from build123d import *

# Parameters (mm, degrees)
SKETCH1_W           = 558.8
SKETCH1_H           = 368.6625
SKETCH1_W_2         = 552.45
SKETCH1_H_2         = 362.3125
SKETCH1_W_3         = 3.175
SKETCH1_W_4         = 89.789
SKETCH1_W_5         = 89.15625
SKETCH1_W_6         = 88.26275
BOSS_EXTRUDE1_DEPTH = 3.175
SKETCH2_W           = 558.8
SKETCH2_H           = 368.6625
SKETCH2_W_2         = 552.45
SKETCH2_H_2         = 362.3125
SKETCH2_W_3         = 3.175
BOSS_EXTRUDE2_DEPTH = 162.9
SKETCH3_W           = 558.8
SKETCH3_H           = 368.6625
BOSS_EXTRUDE3_DEPTH = 45
CUT_EXTRUDE1_DEPTH  = 509.457524805
SKETCH5_R           = 3
CUT_EXTRUDE2_DEPTH  = 509.457524805
LPATTERN1_COUNT     = 3
LPATTERN1_PITCH     = 185.928
SKETCH6_R           = 3
CUT_EXTRUDE3_DEPTH  = 509.457524805
LPATTERN2_COUNT     = 2
LPATTERN2_PITCH     = 185.928


with BuildPart() as part:
    # Sketch1 → Boss-Extrude1 (new body)
    # profile 1 of 12: a face of its own
    with BuildSketch(Plane.XY):
        Rectangle(SKETCH1_W, SKETCH1_H)
        Rectangle(SKETCH1_W_2, SKETCH1_H_2, mode=Mode.SUBTRACT)
    # profile 2 of 12: a face of its own
    with BuildSketch(Plane.XY):
        with Locations((-185.48125, 0)):
            Rectangle(SKETCH1_W_3, SKETCH1_H_2)
    # profile 3 of 12: a face of its own
    with BuildSketch(Plane.XY):
        with Locations((-138.99925, 0)):
            Rectangle(SKETCH1_W_4, SKETCH1_H_2)
    # profile 4 of 12: a face of its own
    with BuildSketch(Plane.XY):
        with Locations((-231.646875, 0)):
            Rectangle(SKETCH1_W_5, SKETCH1_H_2)
    # profile 5 of 12: a face of its own
    with BuildSketch(Plane.XY):
        with Locations((-46.03525, 0)):
            Rectangle(SKETCH1_W_4, SKETCH1_H_2)
    # profile 6 of 12: a face of its own
    with BuildSketch(Plane.XY):
        with Locations((-92.51725, 0)):
            Rectangle(SKETCH1_W_3, SKETCH1_H_2)
    # profile 7 of 12: a face of its own
    with BuildSketch(Plane.XY):
        with Locations((46.92875, 0)):
            Rectangle(SKETCH1_W_4, SKETCH1_H_2)
    # profile 8 of 12: a face of its own
    with BuildSketch(Plane.XY):
        with Locations((0.44675, 0)):
            Rectangle(SKETCH1_W_3, SKETCH1_H_2)
    # profile 9 of 12: a face of its own
    with BuildSketch(Plane.XY):
        with Locations((139.89275, 0)):
            Rectangle(SKETCH1_W_4, SKETCH1_H_2)
    # profile 10 of 12: a face of its own
    with BuildSketch(Plane.XY):
        with Locations((93.41075, 0)):
            Rectangle(SKETCH1_W_3, SKETCH1_H_2)
    # profile 11 of 12: a face of its own
    with BuildSketch(Plane.XY):
        with Locations((232.093625, 0)):
            Rectangle(SKETCH1_W_6, SKETCH1_H_2)
    # profile 12 of 12: a face of its own
    with BuildSketch(Plane.XY):
        with Locations((186.37475, 0)):
            Rectangle(SKETCH1_W_3, SKETCH1_H_2)
    extrude(amount=BOSS_EXTRUDE1_DEPTH)

    # Sketch2 → Boss-Extrude2 (add)
    # profile 1 of 6: a face of its own
    with BuildSketch(Plane.XY.offset(3.175)):
        Rectangle(SKETCH2_W, SKETCH2_H)
        Rectangle(SKETCH2_W_2, SKETCH2_H_2, mode=Mode.SUBTRACT)
    # profile 2 of 6: a face of its own
    with BuildSketch(Plane.XY.offset(3.175)):
        with Locations((-185.48125, 0)):
            Rectangle(SKETCH2_W_3, SKETCH2_H_2)
    # profile 3 of 6: a face of its own
    with BuildSketch(Plane.XY.offset(3.175)):
        with Locations((-92.51725, 0)):
            Rectangle(SKETCH2_W_3, SKETCH2_H_2)
    # profile 4 of 6: a face of its own
    with BuildSketch(Plane.XY.offset(3.175)):
        with Locations((0.44675, 0)):
            Rectangle(SKETCH2_W_3, SKETCH2_H_2)
    # profile 5 of 6: a face of its own
    with BuildSketch(Plane.XY.offset(3.175)):
        with Locations((93.41075, 0)):
            Rectangle(SKETCH2_W_3, SKETCH2_H_2)
    # profile 6 of 6: a face of its own
    with BuildSketch(Plane.XY.offset(3.175)):
        with Locations((186.37475, 0)):
            Rectangle(SKETCH2_W_3, SKETCH2_H_2)
    extrude(amount=BOSS_EXTRUDE2_DEPTH)

    # Sketch3 → Boss-Extrude3 (add)
    with BuildSketch(Plane.XY.offset(166.075)):
        Rectangle(SKETCH3_W, SKETCH3_H)
        Polygon((187.96225, 181.15625), (276.225, 181.15625), (276.225, -181.15625), (187.96225, -181.15625), (184.78725, -181.15625), (94.99825, -181.15625), (91.82325, -181.15625), (2.03425, -181.15625), (-1.14075, -181.15625), (-90.92975, -181.15625), (-94.10475, -181.15625), (-183.89375, -181.15625), (-187.06875, -181.15625), (-276.225, -181.15625), (-276.225, 181.15625), (-187.06875, 181.15625), (-183.89375, 181.15625), (-94.10475, 181.15625), (-90.92975, 181.15625), (-1.14075, 181.15625), (2.03425, 181.15625), (91.82325, 181.15625), (94.99825, 181.15625), (184.78725, 181.15625), align=None, mode=Mode.SUBTRACT)
    extrude(amount=BOSS_EXTRUDE3_DEPTH)

    # Sketch4 → Cut-Extrude1 (cut, through all)
    with BuildSketch(Plane.XZ.offset(184.33125)):
        Polygon((279.4, 211.075), (209.4, 211.075), (279.4, 151.075), align=None)
    extrude(amount=-CUT_EXTRUDE1_DEPTH, mode=Mode.SUBTRACT)

    # Sketch5 → Cut-Extrude2 (cut, through all)
    with BuildSketch(Plane.XZ.offset(184.33125)):
        with Locations(Location((-210.146875, 12.7, 0), (0, 0, 270))):
            Circle(SKETCH5_R)
        with Locations(Location((-245.146875, 12.7, 0), (0, 0, 270))):
            Circle(SKETCH5_R)
        with Locations(Location((-210.146875, 132.7, 0), (0, 0, 270))):
            Circle(SKETCH5_R)
        with Locations(Location((-245.146875, 132.7, 0), (0, 0, 270))):
            Circle(SKETCH5_R)
    cut_extrude2 = extrude(amount=-CUT_EXTRUDE2_DEPTH, mode=Mode.SUBTRACT)

    # LPattern1: Cut-Extrude2 ×3
    with Locations(*[(i * LPATTERN1_PITCH, 0, 0) for i in range(1, LPATTERN1_COUNT)]):
        add(cut_extrude2, mode=Mode.SUBTRACT)

    # Sketch6 → Cut-Extrude3 (cut, through all)
    with BuildSketch(Plane.XZ.offset(184.33125)):
        with Locations(Location((-125.49925, 132.7, 0), (0, 0, 270))):
            Circle(SKETCH6_R)
        with Locations(Location((-160.49925, 132.7, 0), (0, 0, 270))):
            Circle(SKETCH6_R)
        with Locations(Location((-125.49925, 12.7, 0), (0, 0, 270))):
            Circle(SKETCH6_R)
        with Locations(Location((-160.49925, 12.7, 0), (0, 0, 270))):
            Circle(SKETCH6_R)
    cut_extrude3 = extrude(amount=-CUT_EXTRUDE3_DEPTH, mode=Mode.SUBTRACT)

    # LPattern2: Cut-Extrude3 ×2
    with Locations(*[(i * LPATTERN2_PITCH, 0, 0) for i in range(1, LPATTERN2_COUNT)]):
        add(cut_extrude3, mode=Mode.SUBTRACT)


solid = part.part
Work out the finished part from the listing and answer in its coordinate system (mm). A direction names the side the tool comes from. Coordinates: 2 decimals unless noted, no trailing zeros. Order: outer loops, then holes, each group sorted by start corner. A loop starts at its lowest first (then second) coordinate and runs counter-clockwise, first axis right, second up. Notation, with made-up numbers: (-37.75, 14) - (-12.75, 14) arc R22 ccw to (-12.75, 50) - close; hole circle Ø5 at (37, 21.25). An arc over 180 degrees is marked (long way). Put each result on its own line as item: value. Start each with the question number.
1) Find section A-A (z = 123). Give the vertices of the cut face in (x, y) (3 decimals).
2) Find section C-C (x = -149.5). Give the vertices of the cut face in (y, z) (3 decimals).
3) Flat-ended cylindrical pins translate along their axes: pin 1 (6 mm diameter, centred on x = -156.5, y = -118, fed in from -Z); pin 2 (5.5 mm diameter, centred on x = 126.71, z = 12.7, fed in from -Y); pin 3 (3.5 mm diameter, centred on x = -0.5, y = 22, fed in from +Z) (3 decimals). Find the tip coordinate at first contact, or state that the pin passes through.
4) Find section B-B (y = 29). Give the vertices of the cut face in (x, z) (3 decimals), plus the area to 3 significant figures.
5) Find the intervals of material crossed by line 1 (Y direction, x = 12, z = 139.5); line 2 (Z direction, x = -185, y = 122.5) (3 decimals); line 3 (Z direction, x = -251.5, y = -137) (3 decimals), in increasing order. Write a range as from..to.
6) For faces 4 (the flat face through (-90.93, -3, 83)), 5 (the flat face through (277.94, -0.86, 152.326)), determine the directions among +Z, -Z, +X, -X, +Y, -Y from which every point of the face is accessible in a straight line to the end or side of a thin tool.
7) For a pull along Y with two mould halves and no side action, classify faces 1 (the flat face through (-4, -184.331, 104)), 2 (the flat face through (-4, 181.156, 106)), 3 (the flat face through (-279.4, -3, 104)) as released by +Y, released by -Y, zero draft, split by the parting line, or undercut.
Results list:
1. outline: (-279.4, -184.331) - (279.4, -184.331) - (279.4, 184.331) - (-279.4, 184.331) - close; hole (-276.225, -181.156) - (-187.069, -181.156) - (-187.069, 181.156) - (-276.225, 181.156) - close; hole (-183.894, -181.156) - (-94.105, -181.156) - (-94.105, 181.156) - (-183.894, 181.156) - close; hole (-90.93, -181.156) - (-1.141, -181.156) - (-1.141, 181.156) - (-90.93, 181.156) - close; hole (2.034, -181.156) - (91.823, -181.156) - (91.823, 181.156) - (2.034, 181.156) - close; hole (94.998, -181.156) - (184.787, -181.156) - (184.787, 181.156) - (94.998, 181.156) - close; hole (187.962, -181.156) - (276.225, -181.156) - (276.225, 181.156) - (187.962, 181.156) - close
2. outline: (-184.331, 0) - (184.331, 0) - (184.331, 211.075) - (181.156, 211.075) - (181.156, 3.175) - (-181.156, 3.175) - (-181.156, 211.075) - (-184.331, 211.075) - close
3. pin 1: stops at z = 0
3. pin 2: passes through
3. pin 3: stops at z = 166.075
4. outline: (-279.4, 0) - (279.4, 0) - (279.4, 151.075) - (276.225, 153.796) - (276.225, 3.175) - (187.962, 3.175) - (187.962, 166.075) - (184.787, 166.075) - (184.787, 3.175) - (94.998, 3.175) - (94.998, 166.075) - (91.823, 166.075) - (91.823, 3.175) - (2.034, 3.175) - (2.034, 166.075) - (-1.141, 166.075) - (-1.141, 3.175) - (-90.93, 3.175) - (-90.93, 166.075) - (-94.105, 166.075) - (-94.105, 3.175) - (-183.894, 3.175) - (-183.894, 166.075) - (-187.069, 166.075) - (-187.069, 3.175) - (-276.225, 3.175) - (-276.225, 211.075) - (-279.4, 211.075) - close
4. area: 5,490 mm^2
5. line 1: y = -184.33..-181.16, 181.16..184.33
5. line 2: z = 0..166.075
5. line 3: z = 0..3.175
6. face 4: +Z
6. face 5: +Z, +X, +Y, -Y
7. face 1: released by -Y
7. face 2: undercut
7. face 3: zero draft
